from build123d import *

# Parameters (mm, degrees)
BOSS_EXTRUDE1_START     = -317.5
SKETCH4_R               = 2.54
SKETCH4_R_2             = 9.525
SKETCH4_R_3             = 14.2875
BOSS_EXTRUDE1_DEPTH     = 3.175
BOSS_EXTRUDE2_DEPTH     = 3.175
BOSS_EXTRUDE3_START     = -76.2
BOSS_EXTRUDE3_DEPTH     = 3.175
SKETCH9_R               = 2.54
CUT_EXTRUDE2_DEPTH      = 506.024067921
LPATTERN1_COUNT         = 10
LPATTERN1_PITCH         = 50.8
BOSS_EXTRUDE4_START     = 12.7
SKETCH10_R              = 2.54
BOSS_EXTRUDE4_DEPTH     = 12.7
CUT_EXTRUDE3_START      = -76.2
SKETCH11_W              = 25.4
SKETCH11_H              = 725.706439768
SKETCH11_R              = 2.54
SKETCH11_W_2            = 44.268323152
CUT_EXTRUDE3_DEPTH      = 76.2
SKETCH17_R              = 2.54
CUT_EXTRUDE7_DEPTH      = 641.418199343
CIRPATTERN1_COUNT       = 15
CIRPATTERN1_ANGLE       = 210
BOSS_EXTRUDE6_START     = 25.4
SKETCH18_R              = 482.6
SKETCH18_R_2            = 444.5
BOSS_EXTRUDE6_DEPTH     = 38.1
BOSS_EXTRUDE7_START     = 101.6
BOSS_EXTRUDE7_DEPTH     = 6.35
SKETCH17_2_R            = 2.54
CUT_EXTRUDE8_DEPTH      = 691.983880058
CIRPATTERN2_COUNT       = 15
CIRPATTERN2_ANGLE       = 210
CUT_EXTRUDE9_DEPTH      = 50.8
CUT_EXTRUDE9_DEPTH_BACK = 691.983880058
SKETCH21_R              = 848.891258833
SKETCH25_R              = 608.013624822
CUT_EXTRUDE12_DEPTH     = 127


with BuildPart() as part:
    # Sketch4 → Boss-Extrude1 (new body)
    with BuildSketch(Plane(origin=(0, 0, 0), x_dir=(0, 0, -1), z_dir=(1, 0, 0)).offset(BOSS_EXTRUDE1_START)):
        with BuildLine():
            Line((362.853219884, 88.9), (0, 88.9))
            Line((0, 88.9), (0, 65.0875))
            ThreePointArc((0, 65.0875), (14.2875, 50.8), (0, 36.5125))
            Line((0, 36.5125), (0, 12.7))
            Line((0, 12.7), (362.853219884, 12.7))
            Line((362.853219884, 12.7), (362.853219884, 88.9))
        make_face()
        with Locations((53.34, 25.4)):
            Circle(SKETCH4_R, mode=Mode.SUBTRACT)
        with Locations((53.34, 50.8)):
            Circle(SKETCH4_R_2, mode=Mode.SUBTRACT)
        with Locations((177.45964, 50.8)):
            Circle(SKETCH4_R_3, mode=Mode.SUBTRACT)
        with Locations((53.34, 76.2)):
            Circle(SKETCH4_R, mode=Mode.SUBTRACT)
        with Locations((337.453219884, 53.975)):
            Circle(SKETCH4_R_3, mode=Mode.SUBTRACT)
    extrude(amount=-BOSS_EXTRUDE1_DEPTH)

    # Sketch7 → Boss-Extrude2 (add)
    with BuildSketch(Plane(origin=(0, 88.9, 0), x_dir=(1, 0, 0), z_dir=(0, 1, 0))):
        Polygon((-319.0875, 0), (-342.9, 0), (-342.9, 362.853219884), (-317.5, 362.853219884), align=None)
    extrude(amount=-BOSS_EXTRUDE2_DEPTH)

    # Sketch7<2> → Boss-Extrude3 (add)
    with BuildSketch(Plane(origin=(0, 88.9, 0), x_dir=(1, 0, 0), z_dir=(0, 1, 0)).offset(BOSS_EXTRUDE3_START)):
        Polygon((-319.0875, 0), (-342.9, 0), (-342.9, 362.853219884), (-317.5, 362.853219884), align=None)
    extrude(amount=BOSS_EXTRUDE3_DEPTH)

    # Sketch9 → Cut-Extrude2 (cut, through all)
    with BuildSketch(Plane(origin=(0, 88.9, 0), x_dir=(1, 0, 0), z_dir=(0, 1, 0))):
        with Locations(Location((-330.2, 355.6, 0), (0, 0, 270))):
            Circle(SKETCH9_R)
    cut_extrude2 = extrude(amount=-CUT_EXTRUDE2_DEPTH, mode=Mode.SUBTRACT)

    # LPattern1: Cut-Extrude2 ×10
    with Locations(*[(0, 0, i * LPATTERN1_PITCH) for i in range(1, LPATTERN1_COUNT)]):
        add(cut_extrude2, mode=Mode.SUBTRACT)

    # Mirror1: part across face


with BuildPart() as part_1:
    add(part.part)
    add(part.part.mirror(Plane(origin=(-320.239664948, 22.265914948, 0), x_dir=(1, 0, 0), z_dir=(0, 0, 1))))

    # Sketch10 → Boss-Extrude4 (add)
    with BuildSketch(Plane(origin=(0, 88.9, 0), x_dir=(1, 0, 0), z_dir=(0, 1, 0)).offset(BOSS_EXTRUDE4_START)):
        with BuildLine():
            Line((0, -452.755), (0, 452.755))
            ThreePointArc((0, 452.755), (-233.269031744, 388.03691687), (-399.849790193, 212.38464))
            Line((-399.849790193, 212.38464), (-381, 212.38464))
            Line((-381, 212.38464), (-381, 142.53464))
            Line((-381, 142.53464), (-419.1, 142.53464))
            Line((-419.1, 142.53464), (-419.1, 171.295884437))
            ThreePointArc((-419.1, 171.295884437), (-452.755, 0), (-419.1, -171.295884437))
            Line((-419.1, -171.295884437), (-419.1, -142.53464))
            Line((-419.1, -142.53464), (-381, -142.53464))
            Line((-381, -142.53464), (-381, -212.38464))
            Line((-381, -212.38464), (-399.849790193, -212.38464))
            ThreePointArc((-399.849790193, -212.38464), (-356.378451147, -279.251659947), (-301.848330151, -337.453219884))
            ThreePointArc((-301.848330151, -337.453219884), (-161.560294405, -422.948414463), (0, -452.755))
        make_face()
        with Locations(Location((-330.2, -304.8, 0), (0, 0, 90))):
            Circle(SKETCH10_R, mode=Mode.SUBTRACT)
        with Locations(Location((-330.2, -254, 0), (0, 0, 90))):
            Circle(SKETCH10_R, mode=Mode.SUBTRACT)
        with Locations(Location((-330.2, -203.2, 0), (0, 0, 90))):
            Circle(SKETCH10_R, mode=Mode.SUBTRACT)
        with Locations(Location((-330.2, -152.4, 0), (0, 0, 90))):
            Circle(SKETCH10_R, mode=Mode.SUBTRACT)
        with Locations(Location((-330.2, -101.6, 0), (0, 0, 90))):
            Circle(SKETCH10_R, mode=Mode.SUBTRACT)
        with Locations(Location((-330.2, -50.8, 0), (0, 0, 90))):
            Circle(SKETCH10_R, mode=Mode.SUBTRACT)
        with Locations(Location((-330.2, 0, 0), (0, 0, 270))):
            Circle(SKETCH10_R, mode=Mode.SUBTRACT)
        with Locations(Location((-330.2, 50.8, 0), (0, 0, 270))):
            Circle(SKETCH10_R, mode=Mode.SUBTRACT)
        with Locations(Location((-330.2, 101.6, 0), (0, 0, 270))):
            Circle(SKETCH10_R, mode=Mode.SUBTRACT)
        with Locations(Location((-330.2, 152.4, 0), (0, 0, 270))):
            Circle(SKETCH10_R, mode=Mode.SUBTRACT)
        with Locations(Location((-330.2, 203.2, 0), (0, 0, 270))):
            Circle(SKETCH10_R, mode=Mode.SUBTRACT)
        with Locations(Location((-330.2, 254, 0), (0, 0, 270))):
            Circle(SKETCH10_R, mode=Mode.SUBTRACT)
        with Locations(Location((-330.2, 304.8, 0), (0, 0, 270))):
            Circle(SKETCH10_R, mode=Mode.SUBTRACT)
        with Locations(Location((-441.325, 88.9, 0), (0, 0, 270))):
            Circle(SKETCH10_R, mode=Mode.SUBTRACT)
        with Locations(Location((-441.325, 0, 0), (0, 0, 270))):
            Circle(SKETCH10_R, mode=Mode.SUBTRACT)
        with Locations(Location((-441.325, -88.9, 0), (0, 0, 270))):
            Circle(SKETCH10_R, mode=Mode.SUBTRACT)
    extrude(amount=-BOSS_EXTRUDE4_DEPTH)

    # Sketch11 → Cut-Extrude3 (cut)
    # profile 1 of 2: a face of its own
    with BuildSketch(Plane.XZ.offset(-12.7).offset(CUT_EXTRUDE3_START)):
        with Locations((-330.2, 0)):
            Rectangle(SKETCH11_W, SKETCH11_H)
        with Locations(Location((-330.2, -203.2, 0), (0, 0, 90))):
            Circle(SKETCH11_R, mode=Mode.SUBTRACT)
        with Locations(Location((-330.2, -101.6, 0), (0, 0, 90))):
            Circle(SKETCH11_R, mode=Mode.SUBTRACT)
        with Locations(Location((-330.2, -304.8, 0), (0, 0, 90))):
            Circle(SKETCH11_R, mode=Mode.SUBTRACT)
        with Locations(Location((-330.2, 203.2, 0), (0, 0, 270))):
            Circle(SKETCH11_R, mode=Mode.SUBTRACT)
        with Locations(Location((-330.2, 101.6, 0), (0, 0, 90))):
            Circle(SKETCH11_R, mode=Mode.SUBTRACT)
        with Locations(Location((-330.2, 304.8, 0), (0, 0, 270))):
            Circle(SKETCH11_R, mode=Mode.SUBTRACT)
        with Locations((-330.2, 355.6)):
            Circle(SKETCH11_R, mode=Mode.SUBTRACT)
        with Locations(Location((-330.2, 50.8, 0), (0, 0, 90))):
            Circle(SKETCH11_R, mode=Mode.SUBTRACT)
        with Locations(Location((-330.2, 152.4, 0), (0, 0, 90))):
            Circle(SKETCH11_R, mode=Mode.SUBTRACT)
        with Locations(Location((-330.2, 254, 0), (0, 0, 270))):
            Circle(SKETCH11_R, mode=Mode.SUBTRACT)
        with Locations((-330.2, -355.6)):
            Circle(SKETCH11_R, mode=Mode.SUBTRACT)
        with Locations(Location((-330.2, -50.8, 0), (0, 0, 90))):
            Circle(SKETCH11_R, mode=Mode.SUBTRACT)
        with Locations(Location((-330.2, -152.4, 0), (0, 0, 90))):
            Circle(SKETCH11_R, mode=Mode.SUBTRACT)
        with Locations(Location((-330.2, -254, 0), (0, 0, 90))):
            Circle(SKETCH11_R, mode=Mode.SUBTRACT)
    # profile 2 of 2: a face of its own
    with BuildSketch(Plane.XZ.offset(-12.7).offset(CUT_EXTRUDE3_START)):
        with Locations((-365.034161576, 0)):
            Rectangle(SKETCH11_W_2, SKETCH11_H)
    extrude(amount=CUT_EXTRUDE3_DEPTH, mode=Mode.SUBTRACT)

    # Sketch17 → Cut-Extrude7 (cut, through all)
    with BuildSketch(Plane(origin=(0, 101.6, 0), x_dir=(1, 0, 0), z_dir=(0, 1, 0))):
        with Locations((0, -410.68625)):
            Circle(SKETCH17_R)
    cut_extrude7 = extrude(amount=-CUT_EXTRUDE7_DEPTH, mode=Mode.SUBTRACT)

    # CirPattern1: Cut-Extrude7 ×15 about axis
    cirpattern1_axis = Axis((0, 0, 0), (0, -1, 0))
    for i in range(1, CIRPATTERN1_COUNT):
        add(cut_extrude7.rotate(cirpattern1_axis, i * CIRPATTERN1_ANGLE / (CIRPATTERN1_COUNT - 1)), mode=Mode.SUBTRACT)

    # Sketch21 → Cut-Extrude9 (cut, two sides: drawn at the far end of the back side and taken through both)
    with BuildSketch(Plane(origin=(0, 101.6, 0), x_dir=(1, 0, 0), z_dir=(0, 1, 0)).offset(-CUT_EXTRUDE9_DEPTH_BACK)):
        Circle(SKETCH21_R)
    extrude(amount=CUT_EXTRUDE9_DEPTH + CUT_EXTRUDE9_DEPTH_BACK, mode=Mode.SUBTRACT)


with BuildPart() as body_2:
    # Sketch18 → Boss-Extrude6 (new body)
    with BuildSketch(Plane(origin=(0, 101.6, 0), x_dir=(1, 0, 0), z_dir=(0, 1, 0)).offset(BOSS_EXTRUDE6_START)):
        with Locations(Location((0, 0, 0), (0, 0, 90))):
            Circle(SKETCH18_R)
        with Locations(Location((0, 0, 0), (0, 0, 90))):
            Circle(SKETCH18_R_2, mode=Mode.SUBTRACT)
    extrude(amount=BOSS_EXTRUDE6_DEPTH)

    # Sketch25 → Cut-Extrude12 (cut)
    with BuildSketch(Plane(origin=(0, 165.1, 0), x_dir=(1, 0, 0), z_dir=(0, 1, 0))):
        Circle(SKETCH25_R)
    extrude(amount=-CUT_EXTRUDE12_DEPTH, mode=Mode.SUBTRACT)


with BuildPart() as body_3:
    # Sketch19 → Boss-Extrude7 (new body)
    with BuildSketch(Plane(origin=(0, 101.6, 0), x_dir=(1, 0, 0), z_dir=(0, 1, 0)).offset(BOSS_EXTRUDE7_START)):
        with BuildLine():
            Line((0, -427.355), (0, -401.955))
            ThreePointArc((0, -401.955), (-401.955, 0), (0, 401.955))
            Line((0, 401.955), (0, 427.355))
            ThreePointArc((0, 427.355), (-427.355, 0), (0, -427.355))
        make_face()
    extrude(amount=BOSS_EXTRUDE7_DEPTH)

    # Sketch17<2> → Cut-Extrude8 (cut, through all)
    with BuildSketch(Plane(origin=(0, 101.6, 0), x_dir=(1, 0, 0), z_dir=(0, 1, 0))):
        with Locations((0, -410.68625)):
            Circle(SKETCH17_2_R)
    cut_extrude8 = extrude(amount=CUT_EXTRUDE8_DEPTH, mode=Mode.SUBTRACT)

    # CirPattern2: Cut-Extrude8 ×15 about axis
    cirpattern2_axis = Axis((0, 0, 0), (0, -1, 0))
    for i in range(1, CIRPATTERN2_COUNT):
        add(cut_extrude8.rotate(cirpattern2_axis, i * CIRPATTERN2_ANGLE / (CIRPATTERN2_COUNT - 1)), mode=Mode.SUBTRACT)


solid = body_3.part
Check sheet for the modelled part. Datum: model origin and axes. Units: mm. Round coordinates to 2 decimals unless told otherwise and drop trailing zeros. Order: outer loops, then holes, each group sorted by start corner. A loop starts at its lowest first (then second) coordinate and runs counter-clockwise, first axis right, second up. Notation, with made-up numbers: M -9.5,68 L 7.5,68 A26 ccw 7.5,85 Z; hole C -12,17.25 d4. An arc over 180 degrees is marked long. One line per item, written item: value. Start each with the question number.
1. Section check B-B on y = 204.5. Give the number of separate pieces and of enclosed holes in the cut face, and give its area (3 significant figures).
2. Section check C-C on x = -263. Enter the section's corners in (y, z).
3. Section check A-A on x = -148. Enter the section's corners in (y, z), and give its area (3 significant figures).
4. Section check D-D on z = 313.5. Enter the section's corners in (x, y).
5. Gauge pin test, flat ends, axial feed: P1, Ø2, axis at y = 205.5, z = 66.5, coming from the -X side; P2, Ø2, axis at x = -202, y = 209, coming from the +Z side; P3, Ø1, axis at y = 204.5, z = 164, coming from the -X side. Record the tip position at first contact, or that the pin passes through.
6. Scan lines: line 1 along X through (y, z) = (206.5, 0) (3 decimals); line 2 along Z through (x, y) = (-155.5, 205); line 3 along Z through (x, y) = (-369, 209). Record each from-to range of solid material in increasing order.
7. Release check for a two-part mould opening along Z. For faces 1 (the cylindrical face through (-401.858, 206.331, 8.839)), 2 (the cylindrical face through (-427.25, 206.33, -9.4)), 3 (the flat face through (-405, 203.2, -2)) record: released by +Z, released by -Z, zero draft, split by the parting line, or undercut.
Results found:
1. separate pieces: 1
1. enclosed holes: 11
1. area: 32,800 mm^2
2. outline: M 203.2,-336.84 L 209.55,-336.84 L 209.55,-303.97 L 203.2,-303.97 Z; M 203.2,303.97 L 209.55,303.97 L 209.55,336.84 L 203.2,336.84 Z
3. outline: M 203.2,-400.91 L 209.55,-400.91 L 209.55,-373.72 L 203.2,-373.72 Z; M 203.2,373.72 L 209.55,373.72 L 209.55,400.91 L 203.2,400.91 Z
3. area: 345 mm^2
4. outline: M -290.43,203.2 L -251.57,203.2 L -251.57,209.55 L -290.43,209.55 Z
5. P1: x = -422.31
5. P2: z = 377.14
5. P3: x = -394.84
6. line 1: -427.355 to -413.226, -408.146 to -401.955
6. line 2: -398.06 to -370.66, 370.66 to 398.06
6. line 3: -215.57 to -159.4, 159.4 to 215.57
7. face 1: undercut
7. face 2: split by the parting line
7. face 3: zero draft
